CAD build for the part. Positions are in the model's coordinates, mm. Face numbers are marked on the shaded views. A direction names the side the tool comes from. Round coordinates to 2 decimals unless told otherwise and drop trailing zeros. Write each loop counter-clockwise with the first axis right and the second up, starting at its lowest first coordinate (ties: lowest second). Pieces come first, ordered by that corner, then holes. Notation, with made-up numbers: (3.25, 60.5) - (49.25, 60.5) arc R23 cw to (49.25, 87.5) - close; hole circle Ø3 at (79, 18.5). An arc over 180 degrees is marked (long way). Put each result on its own line as item: value. Start each with the question number.
Item 1: Cut at C-C (x = -2). Give the cut face in (y, z).
Item 2: Cut at B-B (y = -22.5). Give the cut face in (x, z), and give its area (3 significant figures).
Item 3: Cut at A-A (z = 282.5). Give the cut face in (x, y), and give its area (3 significant figures).
Item 4: Mould opens along X. For the marked faces 1, 2, 3 and 4 say: released by +X, released by -X, zero draft, split by the parting line, or undercut.
Item 5: 3-axis set-ups, long thin cutter, end or side, ignore diameter. For the marked faces 5 and 6: which of +Z, -Z, +X, -X, +Y, -Y reach the whole face in a straight line?
Item 6: Drill centre lines: line 1 (Y direction, x = 10.5, z = 260.5); line 2 (X direction, y = -23, z = 191.5); line 3 (X direction, y = 35, z = 162). Where is each one in solid material? Low to high. Write a range as from..to.
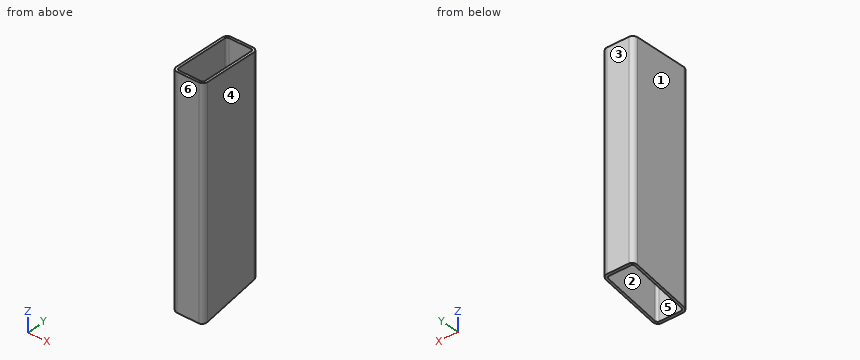
Autodesk Inventor part; units mm, degrees
ref_plane "Start Plane" through (0, 0, 65.051) normal (0, 0, 1) x (1, 0, 0)
ref_plane "End Plane" through (0, 0, 345) normal (0, 0, 1) x (1, 0, 0)
ref_plane "Work Plane4" through (-14, 623.6837, 203.3184) normal (0, 0.2039543, -0.9789804) x (1, 0, 0)
ref_plane "Start Plane" through (0, 0, 65.051) normal (0, 0, 1) x (1, 0, 0)
ref_plane "End Plane" through (0, 0, 345) normal (0, 0, 1) x (1, 0, 0)
sketch "Sketch" plane through (0, 0, 0) normal (0, 0, 1) x (1, 0, 0)
  line L0 (-20, -34) -> (-20, 34)
  line L1 (-14, 40) -> (14, 40)
  line L2 (20, 34) -> (20, -34)
  line L3 (14, -40) -> (-14, -40)
  arc A0 (-20, -34) -> (-14, -40) centre (-14, -34) ccw
  arc A1 (20, 34) -> (14, 40) centre (14, 34) ccw
  arc A2 (-14, 40) -> (-20, 34) centre (-14, 34) ccw
  arc A3 (14, -40) -> (20, -34) centre (14, -34) ccw
  arc A4 (-14, 37) -> (-17, 34) centre (-14, 34) ccw
  line L4 (-14, 37) -> (14, 37)
  arc A5 (17, 34) -> (14, 37) centre (14, 34) ccw
  line L5 (17, 34) -> (17, -34)
  arc A6 (14, -37) -> (17, -34) centre (14, -34) ccw
  line L6 (14, -37) -> (-14, -37)
  arc A7 (-17, -34) -> (-14, -37) centre (-14, -34) ccw
  line L7 (-17, -34) -> (-17, 34)
  line L8 (0, 57.7397) -> (0, -57.7397) construction
  line L9 (-29.7397, 0) -> (29.7397, 0) construction
  dimension "d7" = 6
  dimension "d9" = 40
  dimension "d11" = 80
  dimension "d12" = 3
  dimension "d15" = 20
  dimension "d16" = 40
extrude "Body" add sketch "Sketch" along normal up to surface (279.949 mm away) from surface at 65.051
sketch "Sketch3" plane through (0, 0, 0) normal (0, 0, 1) x (1, 0, 0)
  line L0 (0, 0) -> (10, 0)
ref_plane "Work Plane3" through (0, 0, 0) normal (0, -1, 0) x (1, 0, 0)
ref_plane "Work Plane4" through (-14, 623.6837, 203.3184) normal (0, 0.2039543, -0.9789804) x (1, 0, 0)
split "Split1" plane through (-14, 623.6837, 203.3184) removes the side toward (0, 0.2039543, -0.9789804)
sketch "Sketch4" plane through (0, 0, 0) normal (0, -1, 0) x (1, 0, 0)
  line L0 (-2, 65.051) -> (12, 65.051)
  line L1 (-2, 345) -> (12, 345)
  dimension "d18" = 279.949
equation "\"d7\" = G_IR"
equation "\"d9\" = G_W"
equation "\"d11\" = G_H"
equation "\"d12\" = G_T"
equation "\"d15\" = 0.5 * d9"
equation "\"d16\" = 0.5 * d11"
equation "\"d3\" = G_L"
equation "\"G_W\" = 40"
equation "\"G_H\" = 80"
equation "\"G_T\" = 3"
equation "\"G_IR\" = 6"
equation "\"G_L\" = d18"
equation "\"G_OFFSET_START\" = -65.051"
equation "\"d13\" = -G_OFFSET_START"
equation "\"d14\" = G_OFFSET_END + B_L"
equation "\"B_L\" = 425"
properties part number "ISO 10799-2 - 80x40x3 - 279.95" material "Steel, Mild"
Output values:
1. outline: (-40, 65.05) - (-37, 65.68) - (-37, 345) - (-40, 345) - close; (37, 81.09) - (40, 81.72) - (40, 345) - (37, 345) - close
2. outline: (-20, 68.7) - (-17, 68.7) - (-17, 345) - (-20, 345) - close; (17, 68.7) - (20, 68.7) - (20, 345) - (17, 345) - close
2. area: 1,660 mm2
3. outline: (-20, -34) arc R6 ccw to (-14, -40) - (14, -40) arc R6 ccw to (20, -34) - (20, 34) arc R6 ccw to (14, 40) - (-14, 40) arc R6 ccw to (-20, 34) - close; hole (-17, -34) arc R3 ccw to (-14, -37) - (14, -37) arc R3 ccw to (17, -34) - (17, 34) arc R3 ccw to (14, 37) - (-14, 37) arc R3 ccw to (-17, 34) - close
3. area: 661 mm2
4. face 1: released by -X
4. face 2: undercut
4. face 3: zero draft
4. face 4: released by +X
5. face 5: +Z, -Z
5. face 6: +Z, -Z, +X, -X, -Y
6. line 1: -40..-37, 37..40
6. line 2: -20..-17, 17..20
6. line 3: -19.92..-16.83, 16.83..19.92
